Input: part model. Units: mm. Frame: model coordinates. Coordinates: 2 decimals unless noted, no trailing zeros. Write each loop counter-clockwise with the first axis right and the second up, starting at its lowest first coordinate (ties: lowest second). Pieces come first, ordered by that corner, then holes. Notation, with made-up numbers: M -2,76.25 L 54,76.25 A18 ccw 54,105.25 Z; hole C 43.5,17 d11. An arc over 180 degrees is marked long. Use CSV: the item, a comma, the result in double quotes.
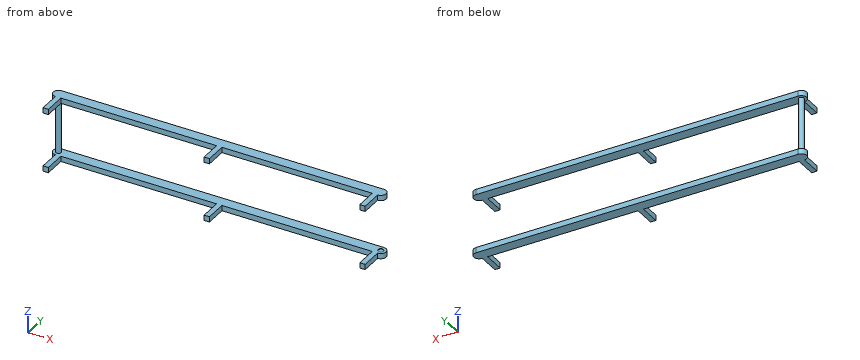
```python
from build123d import *

# Parameters (mm, degrees)
SALIENTE_EXTRUIR1_DEPTH = 10
CROQUIS2_R              = 5
SALIENTE_EXTRUIR2_DEPTH = 100
CROQUIS5_R              = 5
CORTAR_EXTRUIR1_DEPTH   = 1
SALIENTE_EXTRUIR5_DEPTH = 10
CROQUIS7_W              = 10
CROQUIS7_H              = 10
SALIENTE_EXTRUIR6_DEPTH = 40


with BuildPart() as part:
    # Croquis1 → Saliente-Extruir1 (new body)
    with BuildSketch(Plane.XY):
        with BuildLine():
            Line((-300, 10), (300, 10))
            ThreePointArc((300, 10), (310, 0), (300, -10))
            Line((300, -10), (-300, -10))
            ThreePointArc((-300, -10), (-310, 0), (-300, 10))
        make_face()
    extrude(amount=SALIENTE_EXTRUIR1_DEPTH)

    # Croquis2 → Saliente-Extruir2 (add)
    with BuildSketch(Plane.XY.offset(10)):
        with Locations((-300, 0)):
            Circle(CROQUIS2_R)
    extrude(amount=SALIENTE_EXTRUIR2_DEPTH)

    # Croquis5 → Cortar-Extruir1 (cut)
    with BuildSketch(Plane.XY.offset(10)):
        with Locations((300, 0)):
            Circle(CROQUIS5_R)
    extrude(amount=-CORTAR_EXTRUIR1_DEPTH, mode=Mode.SUBTRACT)

    # Croquis6 → Saliente-Extruir5 (add)
    with BuildSketch(Plane.XY.offset(110)):
        with BuildLine():
            Line((-300, -10), (300, -10))
            ThreePointArc((300, -10), (310, 0), (300, 10))
            Line((300, 10), (-300, 10))
            ThreePointArc((-300, 10), (-310, 0), (-300, -10))
        make_face()
    extrude(amount=SALIENTE_EXTRUIR5_DEPTH)

    # Croquis7 → Saliente-Extruir6 (add)
    with BuildSketch(Plane.XZ.offset(10)):
        with Locations((-295, 5)):
            Rectangle(CROQUIS7_W, CROQUIS7_H)
        with Locations((295, 5)):
            Rectangle(CROQUIS7_W, CROQUIS7_H)
        with Locations((295, 115)):
            Rectangle(CROQUIS7_W, CROQUIS7_H)
        with Locations((-295, 115)):
            Rectangle(CROQUIS7_W, CROQUIS7_H)
        with Locations((5, 5)):
            Rectangle(CROQUIS7_W, CROQUIS7_H)
        with Locations((5, 115)):
            Rectangle(CROQUIS7_W, CROQUIS7_H)
    extrude(amount=SALIENTE_EXTRUIR6_DEPTH)


solid = part.part
```
1. Section C-C (z = 40). Return loops of the section in (x, y).
Resolved:
outline,"C -300,0 d10"
2. Section B-B (y = -17.5). Return loops of the section in (x, z), then the cut area to 3 significant figures.
Resolved:
outline,"M -300,0 L -290,0 L -290,10 L -300,10 Z; M -300,110 L -290,110 L -290,120 L -300,120 Z; M 0,0 L 10,0 L 10,10 L 0,10 Z; M 0,110 L 10,110 L 10,120 L 0,120 Z; M 290,0 L 300,0 L 300,10 L 290,10 Z; M 290,110 L 300,110 L 300,120 L 290,120 Z"
area,"600 mm^2"
3. Section A-A (x = 206.5). Return loops of the section in (y, z).
Resolved:
outline,"M -10,0 L 10,0 L 10,10 L -10,10 Z; M -10,110 L 10,110 L 10,120 L -10,120 Z"
4. Contact query for flat-ended pins moving along their axis: pin 1 Ø11 at (x, z) = (-83, 113) entering from -Y; pin 2 Ø8 at (y, z) = (-35, 7) entering from +X; pin 3 Ø11 at (y, z) = (-26.5, 113.5) entering from -X; pin 4 Ø1.5 at (y, z) = (-6, 69.5) entering from +X. Output: stop coordinate, or through.
Resolved:
pin 1,"stops at y = -10"
pin 2,"stops at x = 300"
pin 3,"stops at x = -300"
pin 4,"passes through"
5. Material intervals for line 1 (Z direction, x = -236, y = 0), sorted ascending. Write a range as [from, to].
Resolved:
line 1,"z = [0, 10], [110, 120]"
